```python
from build123d import *

# Parameters (mm, degrees)
SKETCH1_R           = 12.5
BOSS_EXTRUDE1_DEPTH = 4
SKETCH2_R           = 3.7
BOSS_EXTRUDE2_DEPTH = 10


with BuildPart() as part:
    # Sketch1 → Boss-Extrude1 (new body)
    with BuildSketch(Plane(origin=(0, 0, 0), x_dir=(1, 0, 0), z_dir=(0, 1, 0))):
        Circle(SKETCH1_R)
        with BuildLine():
            Line((1.095445115, -1.3), (-1.095445115, -1.3))
            ThreePointArc((-1.095445115, -1.3), (0, 1.7), (1.095445115, -1.3))
        make_face(mode=Mode.SUBTRACT)
    extrude(amount=BOSS_EXTRUDE1_DEPTH)

    # Sketch2 → Boss-Extrude2 (add)
    with BuildSketch(Plane(origin=(0, 4, 0), x_dir=(1, 0, 0), z_dir=(0, 1, 0))):
        Circle(SKETCH2_R)
        with BuildLine():
            Line((-1.095445115, -1.3), (1.095445115, -1.3))
            ThreePointArc((1.095445115, -1.3), (0, 1.7), (-1.095445115, -1.3))
        make_face(mode=Mode.SUBTRACT)
    extrude(amount=BOSS_EXTRUDE2_DEPTH)


solid = part.part
```
The model under review builds one solid part; all positions refer to its coordinate system, in mm. A direction names the side the tool comes from. Round coordinates to 2 decimals unless told otherwise and drop trailing zeros. Loops run counter-clockwise (first coordinate to the right, second up) from the corner with the lowest first, then second, coordinate; pieces in that order, holes last. Notation, with made-up numbers: (77, -32.5) -> (124, -32.5) arc R10 ccw to (124, -17.5) -> close; hole circle Ø10 at (67.25, 76.25). An arc over 180 degrees is marked (long way). Answer as a JSON object with one key per item and string values. Group by question number.
1) For pin 1 Ø3 at (x, z) = (-9, 0) entering from +Y; pin 2 Ø4 at (x, y) = (3.5, 2) entering from +Z; pin 3 Ø6 at (y, z) = (3, -5) entering from -X, all flat-tipped, find the tip position at first contact; note any pin that passes through.
2) We need section A-A on x = 0. Write out the cut boundary in (y, z).
3) For line 1 (X direction, y = 6, z = 0); line 2 (X direction, y = 1.45, z = 0); line 3 (Y direction, x = -2, z = -5.5), list the stretches that pass through material, from the lowest coordinate up. Write a range as [from, to].
4) Mouldability with a two-part tool opening along X and no side actions: class faces 1 (the face through (0, 0, 3)), 2 (the face through (-0.802, 8.93, 3.612)), 3 (the face through (0, 7, 1.3)) as released by +X, released by -X, zero draft, split by the parting line, or undercut.
5) We need section C-C on y = 12.5. Write out the cut boundary in (x, z), then the cut area to 3 significant figures.
6) We need section B-B on z = 0. Write out the cut boundary in (x, y), then the cut area to 3 significant figures.
7) For faces 4 (the face through (0, 14, 2)), 5 (the face through (-3, 4, 3)), list the 3-axis set-ups (+Z, -Z, +X, -X, +Y, -Y) from which the entire face can be reached by the end or side of a thin tool; tool diameter is ignored.
8) We need section D-D on x = -3.25. Write out the cut boundary in (y, z).
Result set:
{
 "1": {"pin 1": "y = 4", "pin 2": "z = 12.41", "pin 3": "x = -12.34"},
 "2": {"outline": "(0, -12.5) -> (4, -12.5) -> (4, -3.7) -> (14, -3.7) -> (14, -1.7) -> (0, -1.7) -> close; (0, 1.3) -> (14, 1.3) -> (14, 3.7) -> (4, 3.7) -> (4, 12.5) -> (0, 12.5) -> close"},
 "3": {"line 1": "[-3.7, -1.7], [1.7, 3.7]", "line 2": "[-12.5, -1.7], [1.7, 12.5]", "line 3": "[0, 4]"},
 "4": {"face 1": "zero draft", "face 2": "split by the parting line", "face 3": "undercut"},
 "5": {"outline": "circle Ø7.4 at (0, 0); hole (-1.1, 1.3) arc R1.7 ccw (long way) to (1.1, 1.3) -> close", "area": "34.5 mm²"},
 "6": {"outline": "(-12.5, 0) -> (-1.7, 0) -> (-1.7, 14) -> (-3.7, 14) -> (-3.7, 4) -> (-12.5, 4) -> close; (1.7, 0) -> (12.5, 0) -> (12.5, 4) -> (3.7, 4) -> (3.7, 14) -> (1.7, 14) -> close", "area": "126 mm²"},
 "7": {"face 4": "+Z, -Z, +X, -X, +Y", "face 5": "+Y"},
 "8": {"outline": "(0, -12.07) -> (4, -12.07) -> (4, -1.77) -> (14, -1.77) -> (14, 1.77) -> (4, 1.77) -> (4, 12.07) -> (0, 12.07) -> close"}
}
